```python
from build123d import *

# Parameters (mm, degrees)
SKETCH1_R           = 14
SKETCH1_R_2         = 9
BOSS_EXTRUDE1_DEPTH = 17.5
SKETCH7_R           = 7.5
SKETCH7_R_2         = 4.5
BOSS_EXTRUDE5_DEPTH = 9.5
BOSS_EXTRUDE7_DEPTH = 2.5
BOSS_EXTRUDE8_DEPTH = 2.5


with BuildPart() as part:
    # Sketch1 → Boss-Extrude1 (new body, symmetric)
    with BuildSketch(Plane.XY):
        Circle(SKETCH1_R)
        Circle(SKETCH1_R_2, mode=Mode.SUBTRACT)
    extrude(amount=BOSS_EXTRUDE1_DEPTH, both=True)



with BuildPart() as body_2:
    # Sketch7 → Boss-Extrude5 (new body, symmetric)
    with BuildSketch(Plane(origin=(0, 0, 0), x_dir=(0, 0, -1), z_dir=(1, 0, 0))):
        with Locations((0, 26)):
            Circle(SKETCH7_R)
        with Locations((0, 26)):
            Circle(SKETCH7_R_2, mode=Mode.SUBTRACT)
    extrude(amount=BOSS_EXTRUDE5_DEPTH, both=True)


with BuildPart() as part_1:
    add(part.part)

    add(body_2.part)  # Boss-Extrude7 merges body 2
    # Sketch8 → Boss-Extrude7 (add, symmetric)
    with BuildSketch(Plane(origin=(0, 0, 0), x_dir=(0, 0, -1), z_dir=(1, 0, 0))):
        with BuildLine():
            Line((-17.5, 14), (-6.153967777, 30.287036342))
            ThreePointArc((-6.153967777, 30.287036342), (0, 18.5), (6.153967777, 30.287036342))
            Line((6.153967777, 30.287036342), (17.5, 14))
            Line((17.5, 14), (17.5, 9))
            Line((17.5, 9), (-17.5, 9))
            Line((-17.5, 9), (-17.5, 14))
        make_face()
    extrude(amount=BOSS_EXTRUDE7_DEPTH, both=True)

    # Sketch9 → Boss-Extrude8 (add, symmetric)
    with BuildSketch(Plane.XY):
        with BuildLine():
            Line((9.5, 18.5), (9.5, 21.5))
            Line((9.5, 21.5), (-9.5, 21.5))
            Line((-9.5, 21.5), (-9.5, 18.5))
            Line((-9.5, 18.5), (-13.514557534, 3.654686672))
            ThreePointArc((-13.514557534, 3.654686672), (0, 14), (13.514557534, 3.654686672))
            Line((13.514557534, 3.654686672), (9.5, 18.5))
        make_face()
    extrude(amount=BOSS_EXTRUDE8_DEPTH, both=True)


solid = part_1.part
```
Source: CAD feature listing. Evaluate the final solid. Frame: model axes, mm. A direction names the side the tool comes from. Round coordinates to 2 decimals unless told otherwise and drop trailing zeros. Loops run counter-clockwise (first coordinate to the right, second up) from the corner with the lowest first, then second, coordinate; pieces in that order, holes last.
1. Section query B-B on x = 0. Output: boundary loops of the cut face in (y, z).
2. Access query for faces 1 (the cylindrical face through (0.133, 33.494, -0.294)), 2 (the flat face through (-7, 14, -2.5)), 3 (the flat face through (7, 15, 2.5)), 4 (the flat face through (2.5, 18, -8)), 5 (the flat face through (-9.5, 26, -5)). Directions: +Z, -Z, +X, -X, +Y, -Y. A direction counts if a zero-diameter tool reaches every point of the face in a straight line with its end or side. Return the directions, or none.
3. Ray query, L1, parallel to Y at x = 3, z = 0; L2, parallel to X at y = 0, z = -2; L3, parallel to Y at x = 0.25, z = 1. Return the intervals inside material, ascending.
4. Mould query, pull axis Y, two halves, no side actions, for faces 6 (the flat face through (-9, 3, 17.5)), 7 (the flat face through (7, 15, -2.5)), 8 (the flat face through (0.035, 22.03, 11.906)). Classes: released by +Y, released by -Y, zero draft, split by the parting line, or undercut.
5. Section query A-A on z = 0. Output: boundary loops of the cut face in (x, y).
6. Section query D-D on z = -5.5. Output: boundary loops of the cut face in (x, y).
7. Contact query for flat-ended pins moving along their axis: pin 1 (16.5 mm diameter, centred on y = 23, z = 0, fed in from -X); pin 2 (7.5 mm diameter, centred on y = 23, z = -9.5, fed in from +X); pin 3 (3 mm diameter, centred on x = -4.5, y = 5.5, fed in from +Z); pin 4 (1 mm diameter, centred on x = -1.5, z = -6, fed in from -Y). Output: stop coordinate, or through.
8. Section query C-C on y = 0. Output: boundary loops of the cut face in (x, z).
Answers below:
1. outline: (-14, -17.5) - (-9, -17.5) - (-9, 17.5) - (-14, 17.5) - close; (9, -17.5) - (14, -17.5) - (30.29, -6.15) arc R7.5 ccw to (30.29, 6.15) - (14, 17.5) - (9, 17.5) - close; hole circle Ø9 at (26, 0)
2. face 1: none
2. face 2: -Z, -X
2. face 3: +Z, +X
2. face 4: -Z, +X
2. face 5: +Z, -Z, -X, +Y
3. L1: y = -13.67 to -8.49, 8.49 to 21.5, 30.5 to 33.5
3. L2: x = -14 to -9, 9 to 14
3. L3: y = -14 to -9, 9 to 21.61, 30.39 to 33.43
4. face 6: zero draft
4. face 7: undercut
4. face 8: released by +Y
5. outline: (-13.51, 3.65) arc R14 ccw (long way) to (13.51, 3.65) - (9.5, 18.5) - (9.5, 21.5) - (-9.5, 21.5) - (-9.5, 18.5) - close; (-9.5, 30.5) - (9.5, 30.5) - (9.5, 33.5) - (-9.5, 33.5) - close; hole circle Ø18 at (0, 0)
6. outline: (-9.5, 20.9) - (-2.5, 20.9) - (-2.5, 13.77) arc R14 ccw (long way) to (2.5, 13.77) - (2.5, 20.9) - (9.5, 20.9) - (9.5, 31.1) - (-9.5, 31.1) - close; hole circle Ø18 at (0, 0)
7. pin 1: stops at x = -10.51
7. pin 2: stops at x = 9.5
7. pin 3: passes through
7. pin 4: stops at y = -13.96
8. outline: (-14, -17.5) - (-9, -17.5) - (-9, 17.5) - (-14, 17.5) - close; (9, -17.5) - (14, -17.5) - (14, 17.5) - (9, 17.5) - close
